Input: part model. Units: mm. Frame: model coordinates. A direction names the side the tool comes from. Coordinates: 2 decimals unless noted, no trailing zeros. Write each loop counter-clockwise with the first axis right and the second up, starting at its lowest first coordinate (ties: lowest second). Pieces come first, ordered by that corner, then holes.
1) Pin query (flat end, axial travel): pin 1 Ø14.5 at (y, z) = (-66.26, -296.22) entering from -X. Return the tip coordinate at first contact, or that it passes through.
2) Section query B-B (z = -88.5). Output: boundary loops of the cut face in (x, y), then the cut area to 3 significant figures.
3) Section query A-A (y = -18). Output: boundary loops of the cut face in (x, z), then the cut area to 3 significant figures.
4) Draft query along X for faces 3 (the cylindrical face through (544.986, -66.499, -290.725)), 4 (the flat face through (544, -70, -211)), 5 (the flat face through (-2, -70, -211)), 6 (the flat face through (546, -68, -211)). Return one class per face: pulls with the +X half, pulls with the -X half, needs draft (parallel to the pull), parting line crosses it, or undercut.
5) Set-up query: faces 1 (the cylindrical face through (-1.014, -117.879, -282.075)), 2 (the flat face through (268, -140, -173)). Return all of +Z, -Z, +X, -X, +Y, -Y with unobstructed straight access to the full face (end or side cutting, diameter ignored); none if empty.
6) Line query: L1, parallel to X at y = -107, z = -209.5; L2, parallel to Y at x = 383, z = -289. Output: solid intervals per line, ascending.
7) Section query D-D (x = 149.5). Output: boundary loops of the cut face in (y, z).
8) Section query C-C (z = -313.5). Output: boundary loops of the cut face in (x, y), then the cut area to 3 significant figures.
from build123d import *

# Parameters (mm, degrees)
TABAN_FLAN_1_DEPTH    = 350
PAH1_SIZE             = 120
IZIM2_R               = 5.5
KES_EKSTR_ZYON1_DEPTH = 614
RADYUS1_R             = 10
RADYUS2_R             = 10
IZIM3_R               = 40
KES_EKSTR_ZYON2_DEPTH = 647
RADYUS3_R             = 20


# Sheet-metal steps are written as plain solids
with BuildPart() as part:
    # Çizim1 → Taban-Flanş1 (new body)
    with BuildSketch(Plane.XY):
        with BuildLine():
            Line((0, 0), (0, -138))
            ThreePointArc((0, -138), (0.585786438, -139.414213562), (2, -140))
            Line((2, -140), (542, -140))
            ThreePointArc((542, -140), (543.414213562, -139.414213562), (544, -138))
            Line((544, -138), (544, 0))
            Line((544, 0), (546, 0))
            Line((546, 0), (546, -138))
            ThreePointArc((546, -138), (544.828427125, -140.828427125), (542, -142))
            Line((542, -142), (2, -142))
            ThreePointArc((2, -142), (-0.828427125, -140.828427125), (-2, -138))
            Line((-2, -138), (-2, 0))
            Line((-2, 0), (0, 0))
        make_face()
    extrude(amount=-TABAN_FLAN_1_DEPTH)

    # Pah1
    pah1_edges = [part.edges().sort_by_distance(p)[0] for p in [
        (-1, 0, 0),
        (545, 0, 0),
    ]]
    chamfer(pah1_edges, length=PAH1_SIZE)

    # Çizim2 → Kes-Ekstrüzyon1 (cut)
    with BuildSketch(Plane.ZY.offset(2)):
        with Locations(Location((-279.118209744, -113.241831987, 0), (0, 0, 180))):
            Circle(IZIM2_R)
        with Locations(Location((-296.219216911, -66.257200948, 0), (0, 0, 180))):
            Circle(IZIM2_R)
    extrude(amount=-KES_EKSTR_ZYON1_DEPTH, mode=Mode.SUBTRACT)

    # Radyus1
    radyus1_edges = [part.edges().sort_by_distance(p)[0] for p in [
        (-1, 0, -350),
        (545, 0, -120),
        (-1, 0, -120),
        (545, 0, -350),
    ]]
    fillet(radyus1_edges, radius=RADYUS1_R)

    # Radyus2
    radyus2_edges = [part.edges().sort_by_distance(p)[0] for p in [
        (545, -120, 0),
        (-1, -120, 0),
    ]]
    fillet(radyus2_edges, radius=RADYUS2_R)

    # Çizim3 → Kes-Ekstrüzyon2 (cut)
    with BuildSketch(Plane.ZY.offset(2)):
        with Locations((-370, -74)):
            Circle(IZIM3_R)
    extrude(amount=-KES_EKSTR_ZYON2_DEPTH, mode=Mode.SUBTRACT)

    # Radyus3
    radyus3_edges = [part.edges().sort_by_distance(p)[0] for p in [
        (545, -39.358983849, -350),
        (545, -108.641016151, -350),
        (-1, -108.641016151, -350),
        (-1, -39.358983849, -350),
    ]]
    fillet(radyus3_edges, radius=RADYUS3_R)


solid = part.part
Answer:
1. pin 1: stops at x = -2
2. outline: (-2, -138) arc R4 ccw to (2, -142) - (542, -142) arc R4 ccw to (546, -138) - (546, -31.5) - (544, -31.5) - (544, -138) arc R2 cw to (542, -140) - (2, -140) arc R2 cw to (0, -138) - (0, -31.5) - (-2, -31.5) - close
2. area: 1,520 mm2
3. outline: (-2, -350) - (0, -350) - (0, -102) - (-2, -102) - close; (544, -350) - (546, -350) - (546, -102) - (544, -102) - close
3. area: 992 mm2
4. face 3: needs draft
4. face 4: undercut
4. face 5: pulls with the -X half
4. face 6: pulls with the +X half
5. face 1: +X, -X
5. face 2: +Z, -Z, +Y
6. L1: x = -2 to 0, 544 to 546
6. L2: y = -142 to -140
7. outline: (-142, -350) - (-140, -350) - (-140, 0) - (-142, 0) - close
8. outline: (-2, -138) arc R4 ccw to (2, -142) - (542, -142) arc R4 ccw to (546, -138) - (546, 0) - (544, 0) - (544, -138) arc R2 cw to (542, -140) - (2, -140) arc R2 cw to (0, -138) - (0, 0) - (-2, 0) - close
8. area: 1,650 mm2
